Part model, mm, in its own coordinate system. Face numbers are marked on the shaded views. A direction names the side the tool comes from. Give positions to 0.01 mm unless a question says otherwise; leave off trailing zeros. Loops run counter-clockwise (first coordinate to the right, second up) from the corner with the lowest first, then second, coordinate; pieces in that order, holes last. Notation, with made-up numbers: (-21, -33.75) -> (16, -33.75) arc R18 cw to (16, -26.75) -> close; hole circle Ø1 at (25.5, 39.5). An arc over 180 degrees is marked (long way). Write item = value, one per line.
from build123d import *

# Parameters (mm, degrees)
EXTRUDE_1_DEPTH           = 9
SHELL_1_T                 = -0.75
SHELL_1_THICKNESS_2_DEPTH = 1.25
CUT_EXTRUDE_1_DEPTH       = 20.602295784
CUT_EXTRUDE_1_DEPTH_BACK  = 20.602295784


with BuildPart() as part:
    # 草图1 → 凸台-拉伸1 (new body)
    with BuildSketch(Plane(origin=(0, 0, 0), x_dir=(1, 0, 0), z_dir=(0, 1, 0))):
        with BuildLine():
            Line((-3.75, 10.34105894), (-3.75, 13.5))
            Line((-3.75, 13.5), (3.75, 13.5))
            Line((3.75, 13.5), (3.75, 10.34105894))
            ThreePointArc((3.75, 10.34105894), (0, -11), (-3.75, 10.34105894))
        make_face()
    extrude(amount=EXTRUDE_1_DEPTH)

    # 抽壳1
    shell_1_openings = [part.faces().sort_by_distance(p)[0] for p in [
        (0, 9, -0.617377205),
    ]]
    offset(amount=SHELL_1_T, openings=shell_1_openings, kind=Kind.INTERSECTION)

    # 抽壳1 thickness 2 face (on inner face of the shell) → 抽壳1 thickness 2 (add)
    with BuildSketch(Plane(origin=(0, 0.75, -0.524637331), x_dir=(0, 0, -1), z_dir=(0, -1, 0))):
        with BuildLine():
            ThreePointArc((9.276510561, -3), (-10.774637331, 0), (9.276510561, 3))
            Line((9.276510561, 3), (12.225362669, 3))
            Line((12.225362669, 3), (12.225362669, -3))
            Line((12.225362669, -3), (9.276510561, -3))
        make_face()
    extrude(amount=-SHELL_1_THICKNESS_2_DEPTH)

    # 草图2 → 切除-拉伸1 (cut, two sides: drawn at the far end of the back side and taken through both)
    with BuildSketch(Plane(origin=(0, 0, 0), x_dir=(0, 0, -1), z_dir=(1, 0, 0)).offset(-CUT_EXTRUDE_1_DEPTH_BACK)):
        Polygon((-6.5, 9), (-5, 4), (6, 4), (7.5, 9), align=None)
    extrude(amount=CUT_EXTRUDE_1_DEPTH + CUT_EXTRUDE_1_DEPTH_BACK, mode=Mode.SUBTRACT)


solid = part.part
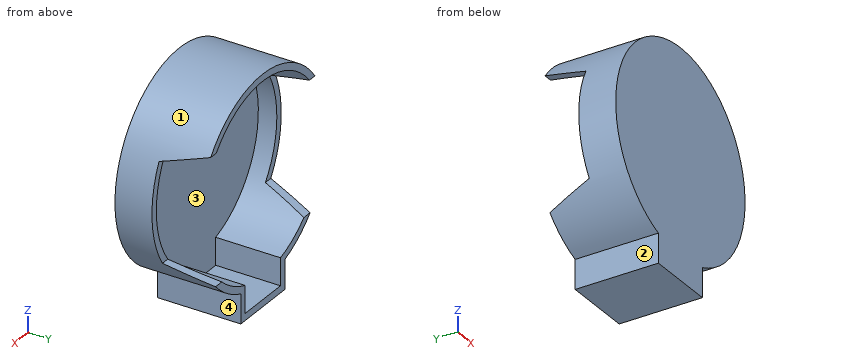
1) Slice it at B-B, the plane x = 0. List the corners of the cut face in (y, z), and give its area (3 significant figures).
Resolved:
outline = (0, -13.5) -> (9, -13.5) -> (9, -12.75) -> (2, -12.75) -> (2, 10.25) -> (9, 10.25) -> (9, 11) -> (0, 11) -> close
area = 59.5 mm²
2) Which spindle directions (+Z, -Z, +X, -X, +Y, -Y) get a long thin tool onto all of the face, cutting with end or side? Do the marked faces 1, 2, 3 and 4. Say none if no direction does.
Resolved:
face_1 = +Y, -Y
face_2 = -Z, -X, +Y, -Y
face_3 = +Y
face_4 = -Z, +X, +Y, -Y
3) Drill centre lines: line 1 along Z through (x, y) = (0, 4); line 2 along X through (y, z) = (3.75, 0); line 3 along X through (y, z) = (0.5, -8.5). Where is each one in solid material? Low to high. Write a range as [from, to].
Resolved:
line_1 = [-13.5, -12.75], [10.25, 11]
line_2 = [-11, -10.25], [10.25, 11]
line_3 = [-6.98, 6.98]
4) Slice it at A-A, the plane y = 5.25. List the corners of the cut face in (x, z) (3 decimals).
Resolved:
outline = (-9.597, 5.375) -> (-8.728, 5.375) arc R10.25 cw to (8.728, 5.375) -> (9.597, 5.375) arc R11 ccw to start; (-8.964, -6.375) arc R11 ccw to (-3.75, -10.341) -> (-3.75, -13.5) -> (3.75, -13.5) -> (3.75, -10.341) arc R11 ccw to (8.964, -6.375) -> (8.026, -6.375) arc R10.25 cw to (3, -9.801) -> (3, -12.75) -> (-3, -12.75) -> (-3, -9.801) arc R10.25 cw to (-8.026, -6.375) -> close
5) Slice it at D-D, the plane y = 7.75. List the corners of the cut face in (x, z) (3 decimals), and give its area (3 significant figures).
Resolved:
outline = (-9.137, 6.125) -> (-8.219, 6.125) arc R10.25 cw to (8.219, 6.125) -> (9.137, 6.125) arc R11 ccw to start; (-8.381, -7.125) arc R11 ccw to (-3.75, -10.341) -> (-3.75, -13.5) -> (3.75, -13.5) -> (3.75, -10.341) arc R11 ccw to (8.381, -7.125) -> (7.369, -7.125) arc R10.25 cw to (3, -9.801) -> (3, -12.75) -> (-3, -12.75) -> (-3, -9.801) arc R10.25 cw to (-7.369, -7.125) -> close
area = 33.0 mm²
6) Drop flat-ended pins along their axis: P1, Ø3, axis at y = 7, z = 8.5, coming from the -X side; P2, Ø8, axis at x = -8, z = -2.5, coming from the -Y side; P3, Ø1.5, axis at y = 6.5, z = -8.5, coming from the +X side; P4, Ø3, axis at y = 6, z = -11, coming from the +X side. Give the stop position or say it passes through.
Resolved:
P1 = -8.49
P2 = 0
P3 = 7.81
P4 = 5.55
7) Slice it at C-C, the plane z = 0. List the corners of the cut face in (x, y), and give its area (3 significant figures).
Resolved:
outline = (-11, 0) -> (11, 0) -> (11, 4) -> (10.25, 4) -> (10.25, 2) -> (-10.25, 2) -> (-10.25, 4) -> (-11, 4) -> close
area = 47.0 mm²
